Work out the finished part from the listing and answer in its coordinate system (mm). Face numbers are marked on the shaded views. A direction names the side the tool comes from. Round coordinates to 2 decimals unless told otherwise and drop trailing zeros. Order: outer loops, then holes, each group sorted by start corner. A loop starts at its lowest first (then second) coordinate and runs counter-clockwise, first axis right, second up. Notation, with made-up numbers: (-25, 85) - (-10, 85) arc R25 ccw to (-10, 122) - close; hole circle Ø11 at (2, -33.5). An arc over 180 degrees is marked (long way). One line per question, with ' | ' between items. Start each with the question number.
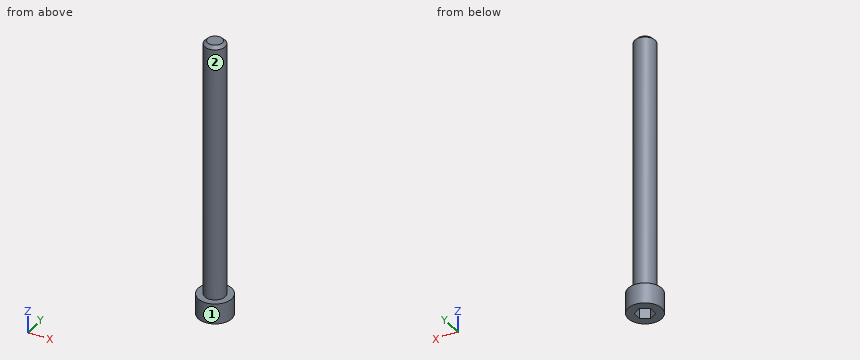
Autodesk Inventor part; units mm, degrees
ref_plane "YZ Plane" through (0, 0, 0) normal (1, 0, 0) x (0, 1, 0)
ref_plane "XZ Plane" through (0, 0, 0) normal (0, 1, 0) x (-1, 0, 0)
ref_plane "XY Plane" through (0, 0, 0) normal (0, 0, 1) x (1, 0, 0)
sketch "Sketch1" plane through (0, 0, 0) normal (0, 0, 1) x (1, 0, 0)
  circle A0 centre (0, 0) radius 1.7526
  dimension "d0" = 3.5052
extrude "Extrusion1" add sketch "Sketch1" along normal blind 44.45
sketch "Sketch2" plane through (0, 0, 0) normal (0, 0, -1) x (-1, 0, 0)
  circle A0 centre (0, 0) radius 1.7526 construction
  circle A1 centre (0, 0) radius 2.8702
  dimension "d3" = 5.7404
extrude "Extrusion2" add sketch "Sketch2" along normal blind 3.5052
sketch "Sketch3" plane through (0, 0, -3.5052) normal (0, 0, -1) x (-1, 0, 0)
  circle A0 centre (0, 0) radius 2.8702
  line L0 (0, 1.604) -> (1.3891, 0.802)
  line L1 (1.3891, 0.802) -> (1.3891, -0.802)
  line L2 (1.3891, -0.802) -> (0, -1.604)
  line L3 (0, -1.604) -> (-1.3891, -0.802)
  line L4 (-1.3891, -0.802) -> (-1.3891, 0.802)
  line L5 (-1.3891, 0.802) -> (0, 1.604)
  dimension "d6" = 2.7781
extrude "Extrusion3" cut sketch "Sketch3" against normal blind 1.7526 contours L0 L1 L2 L3 L4 L5
chamfer "Chamfer1" distance 0.508 angle 45 1 edges at (-1.7526, 0, 44.45)
thread "Thread2"
properties part number "6-32 SHCS x500" material "Stainless Steel"
1) Straight lines are drawn through the part: line 1 (Z direction, x = 0.1, y = 0.8); line 2 (Z direction, x = 0.35, y = 1.8); line 3 (X direction, y = 0.1, z = 11). For each, find the intervals that lie inside material, in ascending order.
2) Section B-B on z = 17.5 is taken. Give the vertices of the cut face in (x, y).
3) Section C-C on x = 2.15 is taken. Give the vertices of the cut face in (y, z), and give its area (3 significant figures).
4) A flat-ended cylindrical pin translates along its axis: pin 1 (2 mm diameter, centred on y = 0, z = 30.5, fed in from -X). Find the tip coordinate at first contact, or state that the pin passes through.
5) For the marked faces 1 and 2, determine the directions among +Z, -Z, +X, -X, +Y, -Y from which every point of the face is accessible in a straight line to the end or side of a thin tool.
6) Section A-A on y = 0 is taken. Give the vertices of the cut face in (x, z), and give its area (3 significant figures).
Recorded:
1) line 1: z = -1.75 to 44.45 | line 2: z = -3.51 to 0 | line 3: x = -1.75 to 1.75
2) outline: circle Ø3.51 at (0, 0)
3) outline: (-1.9, -3.51) - (1.9, -3.51) - (1.9, 0) - (-1.9, 0) - close | area: 13.3 mm²
4) pin 1: stops at x = -1.75
5) face 1: +Z, -Z | face 2: +Z
6) outline: (-2.87, -3.51) - (-1.39, -3.51) - (-1.39, -1.75) - (1.39, -1.75) - (1.39, -3.51) - (2.87, -3.51) - (2.87, 0) - (1.75, 0) - (1.75, 43.94) - (1.24, 44.45) - (-1.24, 44.45) - (-1.75, 43.94) - (-1.75, 0) - (-2.87, 0) - close | area: 171 mm²
